Verification items for this drawing (mm, ordinates from the low corner). A direction names the side the tool comes from. Coordinates: 2 decimals unless noted, no trailing zeros. Loops run counter-clockwise (first coordinate to the right, second up) from the corner with the lowest first, then second, coordinate; pieces in that order, holes last. Notation, with made-up numbers: M -4.5,68.25 L 16.5,68.25 A11 cw 16.5,82.25 Z; hole C 52,-38 d6. An arc over 180 degrees is marked long. Return JSON: item names as keys, results as strings.
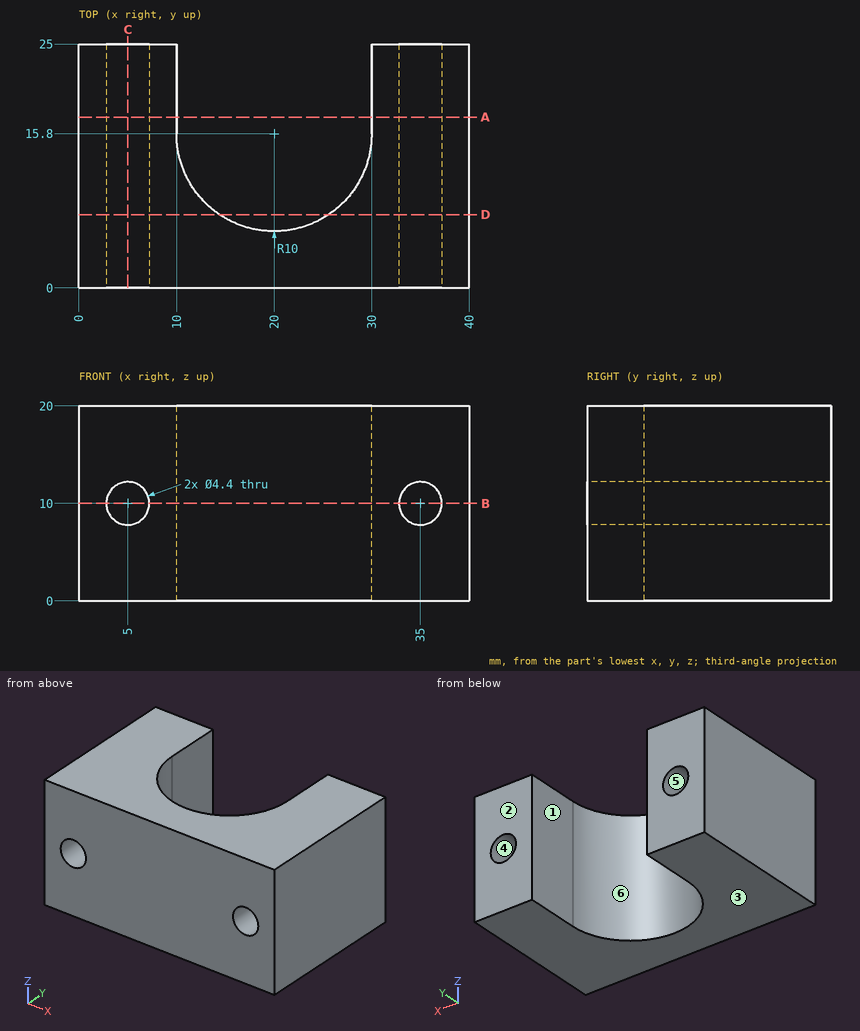
1) Section check C-C on x = 5. Record the cut outline in (y, z), then the cut area to 3 significant figures.
Answers:
{"outline": "M 0,0 L 25,0 L 25,7.8 L 0,7.8 Z; M 0,12.2 L 25,12.2 L 25,20 L 0,20 Z", "area": "390 mm²"}
2) Scan lines: line 1 along Z through (x, y) = (5, 6.25); line 2 along X through (y, z) = (21, 3.25); line 3 along X through (y, z) = (8.5, 4.5). Record each from-to range of solid material in increasing order. Write a range as [from, to].
Answers:
{"line 1": "[0, 7.8], [12.2, 20]", "line 2": "[0, 10], [30, 40]", "line 3": "[0, 13.17], [26.83, 40]"}
3) Set-up check for the marked faces 1 and 2: record each of +Z, -Z, +X, -X, +Y, -Y from which the full face is reachable in a straight line by a thin tool's end or side.
Answers:
{"face 1": "+Z, -Z, +Y", "face 2": "+Z, -Z, +X, -X, +Y"}
4) Section check B-B on z = 10. Record the cut outline in (x, y).
Answers:
{"outline": "M 0,0 L 2.8,0 L 2.8,25 L 0,25 Z; M 7.2,0 L 32.8,0 L 32.8,25 L 30,25 L 30,15.8 A10 cw 10,15.8 L 10,25 L 7.2,25 Z; M 37.2,0 L 40,0 L 40,25 L 37.2,25 Z"}
5) Draft check along Z on the marked faces 3, 4, 5 and 6. Enter one of: +Z half, -Z half, draft (parallel to the pull), parting line (faces both ways), or undercut.
Answers:
{"face 3": "-Z half", "face 4": "undercut", "face 5": "undercut", "face 6": "draft"}
6) Section check A-A on y = 17.5. Record the cut outline in (x, z).
Answers:
{"outline": "M 0,0 L 10,0 L 10,20 L 0,20 Z; M 30,0 L 40,0 L 40,20 L 30,20 Z; hole C 5,10 d4.4; hole C 35,10 d4.4"}
7) Section check D-D on y = 7.5. Record the cut outline in (x, z), then the cut area to 3 significant figures.
Answers:
{"outline": "M 0,0 L 14.42,0 L 14.42,20 L 0,20 Z; M 25.58,0 L 40,0 L 40,20 L 25.58,20 Z; hole C 5,10 d4.4; hole C 35,10 d4.4", "area": "546 mm²"}
